Geometry: final body of the model. Coordinates: model frame, mm. Round coordinates to 2 decimals unless told otherwise and drop trailing zeros. Write each loop counter-clockwise with the first axis right and the second up, starting at its lowest first coordinate (ties: lowest second). Pieces come first, ordered by that corner, then holes.
from build123d import *

# Parameters (mm, degrees)
F1_DEPTH = 15


with BuildPart() as f1:
    # F0 (on Top) → F1 (new body)
    with BuildSketch(Plane.XY):
        with BuildLine():
            ThreePointArc((-21.391129, 20.789386), (-20.512449, 18.668066), (-18.391129, 17.789386))
            Line((-18.391129, 17.789386), (0.608871, 17.789386))
            ThreePointArc((0.608871, 17.789386), (2.730191, 18.668066), (3.608871, 20.789386))
            Line((3.608871, 20.789386), (3.608871, 21.269183))
            ThreePointArc((3.608871, 21.269183), (3.49309, 21.736256), (3.172557, 22.095172))
            ThreePointArc((3.172557, 22.095172), (-8.891129, 24.014756), (-20.954815, 22.095172))
            ThreePointArc((-20.954815, 22.095172), (-21.275348, 21.736256), (-21.391129, 21.269183))
            Line((-21.391129, 21.269183), (-21.391129, 20.789386))
        make_face()
    extrude(amount=F1_DEPTH)


solid = f1.part
1) Section C-C on y = 23.25. Output: boundary loops of the cut face in (x, z), plus the area to 3 significant figures.
2) First-contact query: P1, Ø2, axis at x = -0.5, z = 9, coming from the +Y side; P2, Ø1, axis at y = 20, z = 2, coming from the -X side. Flat tips, straight axial feed; report the tip coordinate or a pass-through.
3) Section A-A on z = 13. Output: boundary loops of the cut face in (x, y), plus the area to 3 significant figures.
4) Section B-B on x = -2.25. Output: boundary loops of the cut face in (y, z), plus the area to 3 significant figures.
5) Line query: probe 1 along Y at (x, z) = (-8.5, 2.25); probe 2 along Y at (x, z) = (-12.25, 4.5); probe 3 along X at (y, z) = (21.5, 2). Output: solid intervals per line, ascending.
Filled in:
1. outline: (-16.56, 0) - (-1.22, 0) - (-1.22, 15) - (-16.56, 15) - close
1. area: 230 mm2
2. P1: stops at y = 23.31
2. P2: stops at x = -21.38
3. outline: (-21.39, 20.79) arc R3 ccw to (-18.39, 17.79) - (0.61, 17.79) arc R3 ccw to (3.61, 20.79) - (3.61, 21.27) arc R1 ccw to (3.17, 22.1) arc R38.87 ccw to (-20.95, 22.1) arc R1 ccw to (-21.39, 21.27) - close
3. area: 135 mm2
4. outline: (17.79, 0) - (23.44, 0) - (23.44, 15) - (17.79, 15) - close
4. area: 84.8 mm2
5. probe 1: y = 17.79 to 24.01
5. probe 2: y = 17.79 to 23.87
5. probe 3: x = -21.36 to 3.58
